from build123d import *

# Parameters (mm, degrees)
SKETCH1_W               = 95
SKETCH1_H               = 70
BOSS_EXTRUDE1_DEPTH     = 15
SKETCH2_W               = 60
SKETCH2_H               = 90
CUT_EXTRUDE1_DEPTH      = 5
SKETCH4_W               = 60
SKETCH4_H               = 8
CUT_EXTRUDE2_DEPTH      = 4.45
CUT_REVOLVE_THIN1_START = -30
CUT_REVOLVE_THIN1_DEPTH = 60
SKETCH3_R               = 5
CUT_EXTRUDE3_DEPTH      = 82.891696771
SKETCH6_R               = 4.35
CUT_EXTRUDE4_DEPTH      = 86.914201387


# Read off the part's stored shape, not the designer's step: Cut-Revolve-Thin1
with BuildPart() as part:
    # Sketch1 → Boss-Extrude1 (new body)
    with BuildSketch(Plane(origin=(0, 0, 0), x_dir=(0, 1, 0), z_dir=(0, 0, 1))):
        Rectangle(SKETCH1_W, SKETCH1_H)
    extrude(amount=BOSS_EXTRUDE1_DEPTH)

    # Sketch2 → Cut-Extrude1 (cut)
    with BuildSketch(Plane.XY.offset(15)):
        with Locations((0, -2.5)):
            Rectangle(SKETCH2_W, SKETCH2_H)
    extrude(amount=-CUT_EXTRUDE1_DEPTH, mode=Mode.SUBTRACT)

    # Sketch4 → Cut-Extrude2 (cut)
    with BuildSketch(Plane.XY.offset(10)):
        with Locations((0, -27.5)):
            Rectangle(SKETCH4_W, SKETCH4_H)
    extrude(amount=-CUT_EXTRUDE2_DEPTH, mode=Mode.SUBTRACT)

    # Cut-Revolve-Thin1 outline → Cut-Revolve-Thin1 (cut)
    with BuildSketch(Plane.YZ.offset(CUT_REVOLVE_THIN1_START)):
        with BuildLine():
            Line((-31.5, 5.55), (-31.5, 8.55))
            ThreePointArc((-31.5, 8.55), (-27.5, 0.55), (-23.5, 8.55))
            Line((-23.5, 8.55), (-23.5, 5.55))
            Line((-23.5, 5.55), (-31.5, 5.55))
        make_face()
    extrude(amount=CUT_REVOLVE_THIN1_DEPTH, mode=Mode.SUBTRACT)

    # Sketch3 → Cut-Extrude3 (cut, through all)
    with BuildSketch(Plane(origin=(30, 0, 0), x_dir=(0, -1, 0), z_dir=(-1, 0, 0))):
        with Locations(Location((27.5, 5.546519225, 0), (0, 0, 179.980056627))):
            Circle(SKETCH3_R)
    extrude(amount=-CUT_EXTRUDE3_DEPTH, mode=Mode.SUBTRACT)

    # Sketch6 → Cut-Extrude4 (cut, through all)
    with BuildSketch(Plane(origin=(-35, 0, 0), x_dir=(0, -1, 0), z_dir=(-1, 0, 0))):
        with Locations(Location((27.5, 5.546519225, 0), (0, 0, 90))):
            Circle(SKETCH6_R)
    extrude(amount=-CUT_EXTRUDE4_DEPTH, mode=Mode.SUBTRACT)


solid = part.part
Geometry: final body of the model. Coordinates: model frame, mm. A direction names the side the tool comes from. Round coordinates to 2 decimals unless told otherwise and drop trailing zeros. Loops run counter-clockwise (first coordinate to the right, second up) from the corner with the lowest first, then second, coordinate; pieces in that order, holes last. Notation, with made-up numbers: (44.5, 3) -> (79.5, 3) arc R22 ccw to (79.5, 35) -> close; hole circle Ø9 at (58, 41.25). An arc over 180 degrees is marked (long way). One line per question, with ' | ' between items. Start each with the question number.
1. Section A-A on y = -27.5. Count the separate pieces of the cut face and the enclosed holes in it, and give its area (3 significant figures).
2. Line query: line 1 along Y through (x, z) = (-18, 5.55); line 2 along X through (y, z) = (4, 14); line 3 along Y through (x, z) = (-26, 8.75). Output: solid intervals per line, ascending. Write a range as [from, to].
3. Contact query for flat-ended pins moving along their axis: pin 1 (8 mm diameter, centred on y = -27.5, z = 5.55, fed in from -X); pin 2 (2.5 mm diameter, centred on y = -26.5, z = 2, fed in from +X); pin 3 (2 mm diameter, centred on x = -18.5, y = -33, fed in from +Z); pin 4 (2.5 mm diameter, centred on x = -14, z = 13, fed in from -Y). Output: stop coordinate, or through.
4. Section B-B on x = 26. Output: boundary loops of the cut face in (y, z), and give its area (3 significant figures).
5. Section C-C on y = -10.5. Output: boundary loops of the cut face in (x, z).
6. Set-up query: faces 5 (the face through (31, 7, 15)), 6 (the face through (0, -39, 10)). Return all of +Z, -Z, +X, -X, +Y, -Y with unobstructed straight access to the full face (end or side cutting, diameter ignored); none if empty.
7. Mould query, pull axis Z, two halves, no side actions, for faces 1 (the face through (-0.42, -27.655, 0.552)), 2 (the face through (32.465, -28.586, 10.427)), 3 (the face through (0, -1, 0)), 4 (the face through (30, -3, 12)). Classes: pulls with the +Z half, pulls with the -Z half, needs draft (parallel to the pull), parting line crosses it, or undercut.
Returned:
1) separate pieces: 3 | enclosed holes: 0 | area: 89.5 mm2
2) line 1: y = [-47.5, -32.5], [-22.5, 47.5] | line 2: x = [-35, -30], [30, 35] | line 3: y = [-47.5, -31.5], [-23.5, 47.5]
3) pin 1: passes through | pin 2: stops at x = -30 | pin 3: stops at z = 10 | pin 4: stops at y = 42.5
4) outline: (-47.5, 0) -> (47.5, 0) -> (47.5, 15) -> (42.5, 15) -> (42.5, 10) -> (-23.5, 10) -> (-23.5, 8.55) arc R5 cw (long way) to (-31.5, 8.55) -> (-31.5, 10) -> (-47.5, 10) -> close | area: 896 mm2
5) outline: (-35, 0) -> (35, 0) -> (35, 15) -> (30, 15) -> (30, 10) -> (-30, 10) -> (-30, 15) -> (-35, 15) -> close
6) face 5: +Z, +X, -X, +Y, -Y | face 6: +Z, -Y
7) face 1: undercut | face 2: undercut | face 3: pulls with the -Z half | face 4: needs draft
